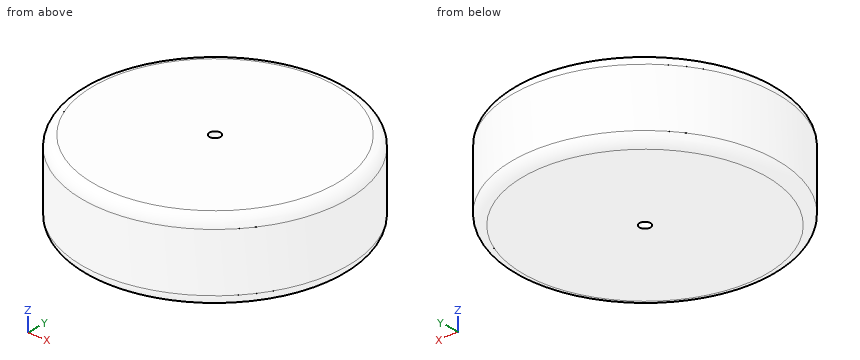
from build123d import *

# Parameters (mm, degrees)
SKETCH1_R           = 25
BOSS_EXTRUDE1_DEPTH = 15
FILLET1_R           = 2
SKETCH7_R           = 1.04
CUT_EXTRUDE2_DEPTH  = 39.405728804


with BuildPart() as part:
    # Sketch1 → Boss-Extrude1 (new body)
    with BuildSketch(Plane.XY):
        Circle(SKETCH1_R)
    extrude(amount=BOSS_EXTRUDE1_DEPTH)

    # Fillet1
    fillet1_edges = [part.edges().sort_by_distance(p)[0] for p in [
        (-25, 0, 0),
        (-25, 0, 15),
    ]]
    fillet(fillet1_edges, radius=FILLET1_R)

    # Sketch7 → Cut-Extrude2 (cut, through all)
    with BuildSketch(Plane.XY.offset(15)):
        Circle(SKETCH7_R)
    extrude(amount=-CUT_EXTRUDE2_DEPTH, mode=Mode.SUBTRACT)


solid = part.part
Design review of the part built by this model. Coordinates are the model's own, in mm. Round coordinates to 2 decimals unless told otherwise and drop trailing zeros. Order: outer loops, then holes, each group sorted by start corner. A loop starts at its lowest first (then second) coordinate and runs counter-clockwise, first axis right, second up.
1) Consider section A-A (x = 0). State the section outline as (y, z) points, plus the area to 3 significant figures.
The answers:
outline: (-25, 2) arc R2 ccw to (-23, 0) - (-1.04, 0) - (-1.04, 15) - (-23, 15) arc R2 ccw to (-25, 13) - close; (1.04, 0) - (23, 0) arc R2 ccw to (25, 2) - (25, 13) arc R2 ccw to (23, 15) - (1.04, 15) - close
area: 715 mm2
2) Clearance check with flat-ended pins moving along their axes: pin 1 Ø1 at (x, z) = (16, 3) entering from +Y; pin 2 Ø2 at (y, z) = (-3, 6.5) entering from -X; pin 3 Ø4 at (y, z) = (2.5, 11) entering from -X (3 decimals). State where each tip first meets the part, or that it passes through.
The answers:
pin 1: stops at y = 19.62
pin 2: stops at x = -24.92
pin 3: stops at x = -24.995
3) For L1, parallel to Y at x = 0, z = 8; L2, parallel to Y at x = 17, z = 7.75; L3, parallel to X at y = -3, z = 4, list the stretches that pass through material, from the lowest coordinate up.
The answers:
L1: y = -25 to -1.04, 1.04 to 25
L2: y = -18.33 to 18.33
L3: x = -24.82 to 24.82
4) Consider section C-C (z = 8). State the section outline as (x, y) points.
The answers:
outline: circle Ø50 at (0, 0); hole circle Ø2.08 at (0, 0)
